Source: CAD feature listing. Evaluate the final solid. Frame: model axes, mm. A direction names the side the tool comes from. Give positions to 0.01 mm unless a question says otherwise; leave off trailing zeros. Loops run counter-clockwise (first coordinate to the right, second up) from the corner with the lowest first, then second, coordinate; pieces in that order, holes last. Notation, with made-up numbers: (2.5, 33) - (34.5, 33) arc R15 cw to (34.5, 52) - close; hole circle Ø11 at (81.5, -20.5). An arc over 180 degrees is marked (long way). Put each result on its own line as item: value.
```python
from build123d import *

# Parameters (mm, degrees)
SKETCH_1_R          = 10
SKETCH_1_R_2        = 1.5
EXTRUDE_2_DEPTH     = 2.5
SKETCH_2_R          = 3
CUT_EXTRUDE_1_DEPTH = 1
SKETCH_3_R          = 1.5
CUT_EXTRUDE_3_DEPTH = 15.221462653
EXTRUDE_START       = 1.5
SKETCH_4_R          = 4.5
SKETCH_4_R_2        = 3
EXTRUDE_3_DEPTH     = 1.5


with BuildPart() as part:
    # 草图1 → 凸台-拉伸2 (new body)
    with BuildSketch(Plane(origin=(0, 0, 0), x_dir=(1, 0, 0), z_dir=(0, 1, 0))):
        with Locations(Location((0, 0, 0), (0, 0, 270))):
            Circle(SKETCH_1_R)
        with Locations(Location((-5, 5, 0), (0, 0, 270))):
            Circle(SKETCH_1_R_2, mode=Mode.SUBTRACT)
        with Locations(Location((5, 5, 0), (0, 0, 270))):
            Circle(SKETCH_1_R_2, mode=Mode.SUBTRACT)
        with Locations(Location((5, -5, 0), (0, 0, 270))):
            Circle(SKETCH_1_R_2, mode=Mode.SUBTRACT)
        with Locations(Location((-5, -5, 0), (0, 0, 270))):
            Circle(SKETCH_1_R_2, mode=Mode.SUBTRACT)
    extrude(amount=EXTRUDE_2_DEPTH)

    # 草图2 → 切除-拉伸1 (cut)
    with BuildSketch(Plane(origin=(0, 2.5, 0), x_dir=(1, 0, 0), z_dir=(0, 1, 0))):
        with Locations(Location((0, 0, 0), (0, 0, 270))):
            Circle(SKETCH_2_R)
    extrude(amount=-CUT_EXTRUDE_1_DEPTH, mode=Mode.SUBTRACT)

    # 草图3 → 切除-拉伸3 (cut, through all)
    with BuildSketch(Plane(origin=(0, 1.5, 0), x_dir=(1, 0, 0), z_dir=(0, 1, 0))):
        with Locations(Location((0, 0, 0), (0, 0, 270))):
            Circle(SKETCH_3_R)
    extrude(amount=-CUT_EXTRUDE_3_DEPTH, mode=Mode.SUBTRACT)

    # 草图4 → 凸台-拉伸3 (add)
    with BuildSketch(Plane(origin=(0, 2.5, 0), x_dir=(1, 0, 0), z_dir=(0, 1, 0)).offset(EXTRUDE_START)):
        with Locations(Location((0, 0, 0), (0, 0, 270))):
            Circle(SKETCH_4_R)
        with Locations(Location((0, 0, 0), (0, 0, 270))):
            Circle(SKETCH_4_R_2, mode=Mode.SUBTRACT)
    extrude(amount=-EXTRUDE_3_DEPTH)


solid = part.part
```
1) Section query C-C, the plane z = 6. Output: boundary loops of the cut face in (x, y).
Check result:
outline: (-8, 0) - (-6.12, 0) - (-6.12, 2.5) - (-8, 2.5) - close; (-3.88, 0) - (3.88, 0) - (3.88, 2.5) - (-3.88, 2.5) - close; (6.12, 0) - (8, 0) - (8, 2.5) - (6.12, 2.5) - close
2) Pin query (flat end, axial travel): P1, Ø3.5, axis at x = -5, z = 5, coming from the +Y side; P2, Ø1.5, axis at y = 2, z = 2.5, coming from the +X side; P3, Ø1, axis at x = -3, y = 1.5, coming from the -Z side. Return the tip coordinate at first contact, or that it passes through.
Check result:
P1: y = 2.5
P2: x = 9.85
P3: z = -9.68
3) Section query D-D, the plane y = 3.65. Output: boundary loops of the cut face in (x, z).
Check result:
outline: circle Ø9 at (0, 0); hole circle Ø6 at (0, 0)
4) Material intervals for line 1 along X through (y, z) = (2.45, 0); line 2 along X through (y, z) = (1.65, 4.25); line 3 along Y through (x, z) = (7.5, 1.25), sorted ascending. Write a range as [from, to].
Check result:
line 1: [-10, -3], [3, 10]
line 2: [-9.05, -6.3], [-3.7, 3.7], [6.3, 9.05]
line 3: [0, 2.5]
5) Section query A-A, the plane z = 0. Output: boundary loops of the cut face in (x, y), plus the area to 3 significant figures.
Check result:
outline: (-10, 0) - (-1.5, 0) - (-1.5, 1.5) - (-3, 1.5) - (-3, 4) - (-4.5, 4) - (-4.5, 2.5) - (-10, 2.5) - close; (1.5, 0) - (10, 0) - (10, 2.5) - (4.5, 2.5) - (4.5, 4) - (3, 4) - (3, 1.5) - (1.5, 1.5) - close
area: 44.0 mm²
6) Access query for faces 1 (the cylindrical face through (4.425, 1.232, 6.386)), 2 (the flat face through (-1.3, 1.5, 1.3)). Directions: +Z, -Z, +X, -X, +Y, -Y. A direction counts if a zero-diameter tool reaches every point of the face in a straight line with its end or side. Return the directions, or none.
Check result:
face 1: +Y, -Y
face 2: +Y
7) Section query B-B, the plane x = -6. Output: boundary loops of the cut face in (y, z).
Check result:
outline: (0, -8) - (2.5, -8) - (2.5, -6.12) - (0, -6.12) - close; (0, -3.88) - (2.5, -3.88) - (2.5, 3.88) - (0, 3.88) - close; (0, 6.12) - (2.5, 6.12) - (2.5, 8) - (0, 8) - close
8) Mould query, pull axis Z, two halves, no side actions, for faces 3 (the cylindrical face through (-9.76, 1.23, -2.17)), 4 (the flat face through (-3, 4, 1)), 5 (the cylindrical face through (-3.99, 1.23, -6.11)). Classes: pulls with the +Z half, pulls with the -Z half, needs draft (parallel to the pull), parting line crosses it, or undercut.
Check result:
face 3: parting line crosses it
face 4: needs draft
face 5: undercut
